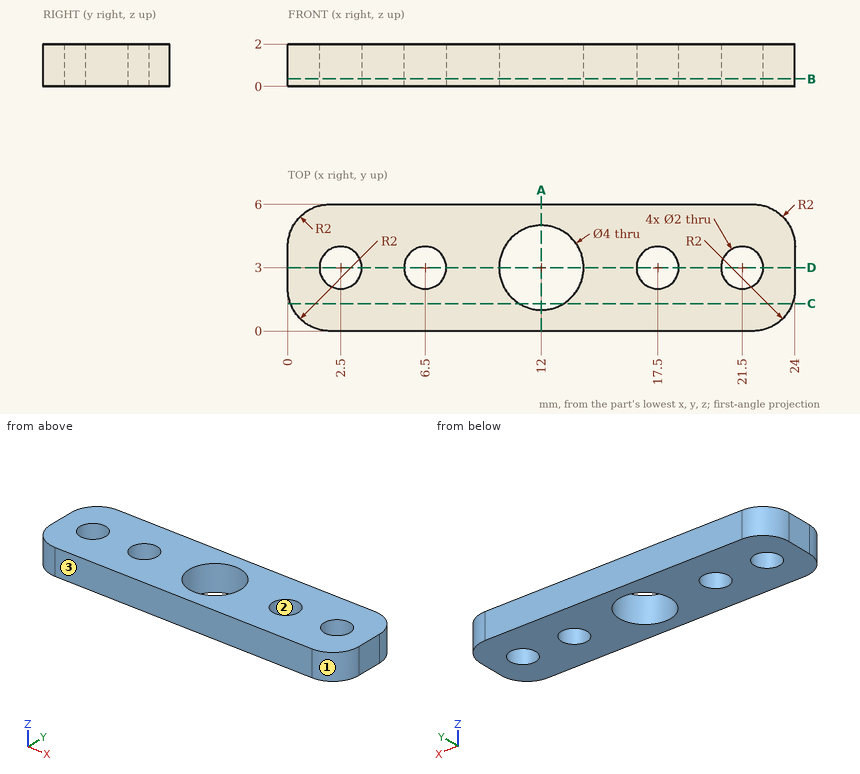
Can you work these out from the drawing? Everything is in mm from the part's minimum corner. Round coordinates to 2 decimals unless told otherwise and drop trailing zeros. Loops run counter-clockwise (first coordinate to the right, second up) from the corner with the lowest first, then second, coordinate; pieces in that order, holes last.
1. If we section it at C-C on y = 1.3: Write out the boundary of the cut face in (x, z), plus the area to 3 significant figures.
Answer list:
outline: (0.13, 0) - (10.95, 0) - (10.95, 2) - (0.13, 2) - close; (13.05, 0) - (23.87, 0) - (23.87, 2) - (13.05, 2) - close
area: 43.3 mm2
2. If we section it at B-B on z = 0.35: Write out the boundary of the cut face in (x, y), plus the area to 3 significant figures.
Answer list:
outline: (0, 2) arc R2 ccw to (2, 0) - (22, 0) arc R2 ccw to (24, 2) - (24, 4) arc R2 ccw to (22, 6) - (2, 6) arc R2 ccw to (0, 4) - close; hole circle Ø2 at (2.5, 3); hole circle Ø2 at (6.5, 3); hole circle Ø4 at (12, 3); hole circle Ø2 at (17.5, 3); hole circle Ø2 at (21.5, 3)
area: 115 mm2
3. If we section it at A-A on x = 12: Write out the boundary of the cut face in (y, z).
Answer list:
outline: (0, 0) - (1, 0) - (1, 2) - (0, 2) - close; (5, 0) - (6, 0) - (6, 2) - (5, 2) - close
4. We'd pull the mould along X, two halves only. Please class the marked faces 1, 2 and 3: +X half, -X half, draft (parallel to the pull), parting line (faces both ways), or undercut.
Answer list:
face 1: +X half
face 2: undercut
face 3: draft
5. If I drill on line 1 along X through (y, z) = (3, 0.5); line 2 along Y through (x, z) = (6.5, 1.3); line 3 along X through (y, z) = (2.65, 1.75), over which ranges is the centre line in solid material (lowest first)?
Answer list:
line 1: x = 0 to 1.5, 3.5 to 5.5, 7.5 to 10, 14 to 16.5, 18.5 to 20.5, 22.5 to 24
line 2: y = 0 to 2, 4 to 6
line 3: x = 0 to 1.56, 3.44 to 5.56, 7.44 to 10.03, 13.97 to 16.56, 18.44 to 20.56, 22.44 to 24
6. If we section it at D-D on y = 3: Write out the boundary of the cut face in (x, z), plus the area to 3 significant figures.
Answer list:
outline: (0, 0) - (1.5, 0) - (1.5, 2) - (0, 2) - close; (3.5, 0) - (5.5, 0) - (5.5, 2) - (3.5, 2) - close; (7.5, 0) - (10, 0) - (10, 2) - (7.5, 2) - close; (14, 0) - (16.5, 0) - (16.5, 2) - (14, 2) - close; (18.5, 0) - (20.5, 0) - (20.5, 2) - (18.5, 2) - close; (22.5, 0) - (24, 0) - (24, 2) - (22.5, 2) - close
area: 24.0 mm2
